Model file for the job. Use its own axes, mm. Face numbers are marked on the shaded views. A direction names the side the tool comes from. Coordinates: 2 decimals unless noted, no trailing zeros. Order: outer loops, then holes, each group sorted by start corner. A loop starts at its lowest first (then second) coordinate and runs counter-clockwise, first axis right, second up. Notation, with made-up numbers: (-0.75, 36.25) -> (14.25, 36.25) arc R7 cw to (14.25, 44.25) -> close; hole circle Ø11 at (-19, -33). An arc over 180 degrees is marked (long way). Write item = value, one per line. Start each with the question number.
Q1. Cut at B-B, the plane z = 14.5. List the corners of the cut face in (x, y).
Q2. Cut at C-C, the plane x = -6. List the corners of the cut face in (y, z).
Q3. Cut at D-D, the plane z = 7.5. List the corners of the cut face in (x, y).
Q4. Flat gauge pins, fed straight in: pin 1 (5 mm diameter, centred on y = -0.5, z = 15, fed in from +X); pin 2 (6 mm diameter, centred on y = 6, z = 27.5, fed in from +X); pin 3 (3 mm diameter, centred on x = 4, y = -1, fed in from -Z). Where does each tip first touch, or does it go through?
Q5. Wall check: line 1 (X direction, y = 0, z = 6.3); line 2 (X direction, y = 0.25, z = 22); line 3 (Z direction, x = -4, y = 0). Give the ranges that are in metal, low to high. Write a range as from..to.
Q6. 3-axis set-ups, long thin cutter, end or side, ignore diameter. For the marked faces 1 and 2: which of +Z, -Z, +X, -X, +Y, -Y reach the whole face in a straight line?
Q7. Cut at A-A, the plane y = 0. List the corners of the cut face in (x, z), plus the area to 3 significant figures.
from build123d import *

# Parameters (mm, degrees)
SKETCH_1_R          = 7.95
EXTRUDE_1_DEPTH     = 30
SKETCH_2_R          = 7.95
EXTRUDE_2_DEPTH     = 10
SKETCH_3_W          = 7.95
SKETCH_3_H          = 15.9
CUT_EXTRUDE_1_DEPTH = 26
SKETCH_4_R          = 2
CUT_EXTRUDE_2_DEPTH = 42.550030084
M3X0_5_1_REACH      = 43.55
M3X0_5_1_BORE_R     = 1.25
CUT_EXTRUDE_3_DEPTH = 39.670466911


with BuildPart() as part:
    # ｽｹｯﾁ1 → ﾎﾞｽ - 押し出し1 (new body)
    with BuildSketch(Plane.XY):
        Circle(SKETCH_1_R)
    extrude(amount=EXTRUDE_1_DEPTH)

    # ｽｹｯﾁ2 → ﾎﾞｽ - 押し出し2 (add)
    with BuildSketch(Plane.XY.offset(30)):
        Circle(SKETCH_2_R)
    extrude(amount=EXTRUDE_2_DEPTH)

    # ｽｹｯﾁ3 → ｶｯﾄ - 押し出し1 (cut)
    with BuildSketch(Plane(origin=(0, 0, 0), x_dir=(-1, 0, 0), z_dir=(0, 0, -1))):
        with Locations((-3.975, 0)):
            Rectangle(SKETCH_3_W, SKETCH_3_H)
    extrude(amount=-CUT_EXTRUDE_1_DEPTH, mode=Mode.SUBTRACT)

    # ｽｹｯﾁ4 → ｶｯﾄ - 押し出し2 (cut, through all)
    with BuildSketch(Plane(origin=(0, 0, 0), x_dir=(0, 0, -1), z_dir=(1, 0, 0))):
        with Locations(Location((-10, 0, 0), (0, 0, 90))):
            Circle(SKETCH_4_R)
    extrude(amount=-CUT_EXTRUDE_2_DEPTH, mode=Mode.SUBTRACT)

    # M3x0.5 ねじ穴1 bore → M3x0.5 ねじ穴1 (cut, up to next)
    with BuildSketch(Plane(origin=(0, 0, 0), x_dir=(-1, 0, 0), z_dir=(0, 0, -1)), mode=Mode.PRIVATE) as m3x0_5_1_sk1:
        with Locations((3.95, 0)):
            Circle(M3X0_5_1_BORE_R)
    m3x0_5_1_tool1 = extrude(m3x0_5_1_sk1.sketch, amount=-M3X0_5_1_REACH, mode=Mode.PRIVATE) & part.part
    add(m3x0_5_1_tool1.solids().sort_by_distance((-3.95, 0, 0))[0], mode=Mode.SUBTRACT)

    # ｽｹｯﾁ7 → ｶｯﾄ - 押し出し3 (cut, through all)
    with BuildSketch(Plane(origin=(0, 0, 3), x_dir=(-1, 0, 0), z_dir=(0, 0, -1))):
        with BuildLine():
            Line((0, 7.95), (0, -7.95))
            ThreePointArc((0, -7.95), (7.95, 0), (0, 7.95))
        make_face()
    extrude(amount=CUT_EXTRUDE_3_DEPTH, mode=Mode.SUBTRACT)


solid = part.part
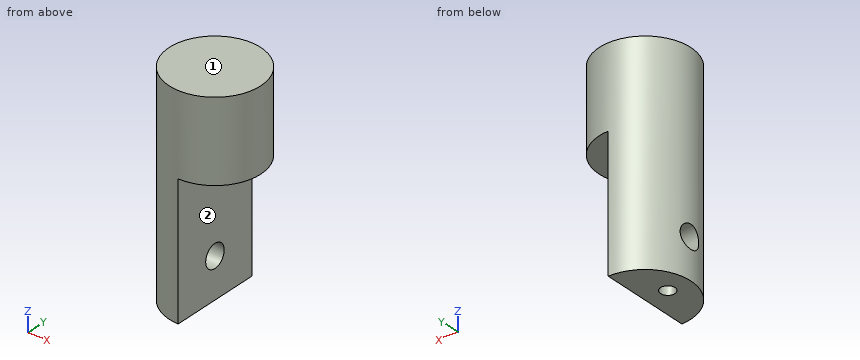
Here are the results:
q1.outline = (0, -7.95) -> (0, 7.95) arc R7.95 ccw to start
q2.outline = (-5.22, 3) -> (5.22, 3) -> (5.22, 40) -> (-5.22, 40) -> close; hole circle Ø4 at (0, 10)
q3.outline = (0, -7.95) -> (0, 7.95) arc R7.95 ccw to start; hole circle Ø2.5 at (-3.95, 0)
q4.pin_1 = 0
q4.pin_2 = 7.36
q4.pin_3 = 26
q5.line_1 = -7.95..-5.2, -2.7..0
q5.line_2 = -7.95..0
q5.line_3 = 12..40
q6.face_1 = +Z, +X, -X, +Y, -Y
q6.face_2 = -Z, +X, +Y, -Y
q7.outline = (-7.95, 3) -> (-5.2, 3) -> (-5.2, 8) -> (-7.95, 8) -> close; (-7.95, 12) -> (0, 12) -> (0, 26) -> (7.95, 26) -> (7.95, 40) -> (-7.95, 40) -> close; (-2.7, 3) -> (0, 3) -> (0, 8) -> (-2.7, 8) -> close
q7.area = 361 mm²
